Input: part model. Units: mm. Frame: model coordinates. Face numbers are marked on the shaded views. A direction names the side the tool comes from. Coordinates: 2 decimals unless noted, no trailing zeros. Loops run counter-clockwise (first coordinate to the right, second up) from the corner with the lowest first, then second, coordinate; pieces in that order, holes last. Notation, with made-up numbers: (74, -34) - (96, -34) arc R20 ccw to (96, -16) - close; hole circle Ø6 at (-19, 75.25). An arc over 180 degrees is marked (long way). Use a Markdown table: item, result. Add a question column.
1. Section query A-A on z = -7. Return the cut outline in (x, y), then the cut area to 3 significant figures.
2. Section query C-C on y = -7.5. Return the cut outline in (x, z).
3. Section query B-B on x = 4. Return the cut outline in (y, z).
4. Draft query along Y for the marked faces 3, 4 and 5. Return one class per face: released by +Y, released by -Y, zero draft, split by the parting line, or undercut.
5. Access query for the marked faces 1 and 2. Directions: +Z, -Z, +X, -X, +Y, -Y. A direction counts if a zero-diameter tool reaches every point of the face in a straight line with its end or side. Return the directions, or none.
6. Section query D-D on x = 16.5. Return the cut outline in (y, z), then the cut area to 3 significant figures.
7. Contact query for flat-ended pins moving along their axis: P1, Ø1.5, axis at x = 1, z = -3.5, coming from the -Y side; P2, Ø1.6, axis at x = 13.5, y = 2, coming from the +Z side; P3, Ø1.2, axis at x = 4, y = -47, coming from the +Z side. Output: stop coordinate, or through.
8. Ray query, L1, parallel to Y at x = 4, z = -4; L2, parallel to Y at x = 10.25, z = -4.5; L3, parallel to X at y = -47, z = -6. Return the intervals inside material, ascending. Write a range as [from, to].
Autodesk Inventor part; units mm, degrees
ref_plane "Płaszczyzna konstrukcyjna1" through (-42.5, -72.5, -8.25) normal (0, 0, 1) x (1, 0, 0)
ref_plane "YZ Plane" through (0, 0, 0) normal (1, 0, 0) x (0, 1, 0)
ref_plane "XZ Plane" through (0, 0, 0) normal (0, 1, 0) x (-1, 0, 0)
sketch "Szkic1" plane through (0, 0, 0) normal (0, 0, 1) x (1, 0, 0)
  line L0 (13.65, -45) -> (17, -45)
  line L1 (0.5, -45) -> (12.85, -45)
  line L2 (17, -25) -> (13.65, -25)
  line L3 (12.85, -25) -> (0.5, -25)
  line L4 (13.65, -20) -> (17, -20)
  line L5 (0.5, -20) -> (12.85, -20)
  line L6 (12.85, 0) -> (0.5, 0)
  line L7 (17, 0) -> (13.65, 0)
  line L8 (0, -25.5) -> (0, -44.5)
  line L9 (0, -0.5) -> (0, -19.5)
  line L10 (17.5, -12.6805) -> (17.5, -0.5)
  line L11 (17.5, -44.5) -> (17.5, -32.3195)
  line L12 (0, -45) -> (17.5, -45)
  line L13 (17.5, -45) -> (17.5, -49)
  line L14 (17.5, -49) -> (0, -49)
  line L15 (0, -49) -> (0, -45)
  line L16 (0, -20) -> (17.5, -20)
  line L17 (17.5, -20) -> (17.5, -25)
  line L18 (17.5, -25) -> (0, -25)
  line L19 (0, -25) -> (0, -20)
  line L20 (0, 0) -> (17.5, 0)
  line L21 (17.5, 0) -> (17.5, 4)
  line L22 (17.5, 4) -> (0, 4)
  line L23 (0, 4) -> (0, 0)
  line L24 (0, 4) -> (17.5, 4)
  line L25 (17.5, 4) -> (17.5, -49)
  line L26 (17.5, -49) -> (0, -49)
  line L27 (0, -49) -> (0, 4)
  dimension "d0" = 4
  dimension "d1" = 4
ref_plane "Płaszczyzna konstrukcyjna1" through (-42.5, -72.5, -8.25) normal (0, 0, 1) x (1, 0, 0)
extrude "Wyciągnięcie proste1" add sketch "Szkic1" against normal up to surface (8.25 mm away) contours L0 L12 L13 L14 L15 L1 | L18 L2 L3 L19 L16 L5 L4 L17 | L20 L7 L6 L23 L22 L21
sketch "Szkic2" plane through (0, 0, 0) normal (0, 0, 1) x (1, 0, 0)
  line L0 (0, 0) -> (17.5, 0)
  line L1 (17.5, 0) -> (17.5, 4)
  line L2 (17.5, 4) -> (0, 4)
  line L3 (0, 4) -> (0, 0)
  line L4 (0, -25) -> (17.5, -25)
  line L5 (17.5, -25) -> (17.5, -20)
  line L6 (17.5, -20) -> (0, -20)
  line L7 (0, -20) -> (0, -25)
  line L8 (0, -49) -> (17.5, -49)
  line L9 (17.5, -49) -> (17.5, -45)
  line L10 (17.5, -45) -> (0, -45)
  line L11 (0, -45) -> (0, -49)
  line L12 (0, 4) -> (17.5, 4)
  line L13 (17.5, 4) -> (0, 4)
  line L14 (0, 4) -> (0, -49)
  line L15 (0, -49) -> (17.5, -49)
  line L16 (17.5, -49) -> (17.5, 4)
extrude "Wyciągnięcie proste2" add sketch "Szkic2" along normal blind 2
sketch "Szkic3" plane through (0, 0, 2) normal (0, 0, 1) x (1, 0, 0)
  line L0 (17.5, -45) -> (0, -45)
  line L1 (0, 4) -> (0, -49)
  line L2 (0, -49) -> (17.5, -49)
  line L3 (17.5, -49) -> (17.5, 4)
  line L4 (0, -25) -> (17.5, -25)
  line L5 (17.5, -20) -> (0, -20)
  line L6 (0, 0) -> (17.5, 0)
  line L7 (17.5, 4) -> (0, 4)
  point P0 (13.5, -47)
  point P1 (4, -47)
  point P2 (13.5, -22.5)
  point P3 (4, -22.5)
  point P4 (13.5, 2)
  point P5 (4, 2)
  dimension "d6" = 2
  dimension "d7" = 2
  dimension "d8" = 2.5
  dimension "d9" = 2.5
  dimension "d10" = 2
  dimension "d11" = 2
  dimension "d12" = 4
  dimension "d13" = 4
  dimension "d14" = 4
  dimension "d15" = 4
  dimension "d16" = 4
  dimension "d17" = 4
hole "Otwór1" at (13.5, -47, 2) at (4, -47, 2) at (13.5, -22.5, 2) at (4, -22.5, 2) at (13.5, 2, 2) at (4, 2, 2) direction (0, 0, -1) diameter 2 end through all
sketch "Szkic4" plane through (0, 0, 2) normal (0, 0, 1) x (1, 0, 0)
  circle A0 centre (13.5, 2) radius 1
  circle A1 centre (13.5, -22.5) radius 1
  circle A2 centre (13.5, -47) radius 1
  circle A3 centre (4, -47) radius 1
  circle A4 centre (4, -22.5) radius 1
  circle A5 centre (4, 2) radius 1
  line L0 (17.5, -49) -> (17.5, 4)
  line L1 (17.5, 4) -> (0, 4)
  line L2 (0, 4) -> (0, -49)
  line L3 (0, -49) -> (17.5, -49)
  point P0 (0, 0)
extrude "Wyciągnięcie proste3" add sketch "Szkic4" against normal blind 3 contours A0 | A1 | A2 | A3 | A4 | A5
fillet "Zaokrąglenie1" radius 5 2 edges at (8.75, 4, 2) (8.75, -49, 2)
sketch "Szkic5" plane through (0, -25, -8.25) normal (-1, 0, 0) x (0, 0, 1)
  arc A0 (5.25, -24) -> (10.25, -19) centre (5.25, -19) ccw
  line L0 (10.25, 24) -> (10.25, -19)
  arc A1 (10.25, 24) -> (5.25, 29) centre (5.25, 24) ccw
  line L1 (0, 29) -> (5.25, 29)
  line L2 (0, 25) -> (0, 29)
  line L3 (8.25, 25) -> (0, 25)
  line L4 (8.25, 25) -> (8.25, 5)
  line L5 (8.25, 5) -> (0, 5)
  line L6 (0, 0) -> (0, 5)
  line L7 (8.25, 0) -> (0, 0)
  line L8 (8.25, 0) -> (8.25, -20)
  line L9 (8.25, -20) -> (0, -20)
  line L10 (0, -24) -> (0, -20)
  line L11 (5.25, -24) -> (0, -24)
  line L12 (0, 25) -> (0, -20)
extrude "Wyciągnięcie proste4" add sketch "Szkic5" along normal blind 1
fillet "Zaokrąglenie2" radius 4 5 edges at (-1, 4, -5.625) (-1, -22.5, 2) (-1, -47.5355, 0.5355) (-1, -49, -5.625) (-1, 2.5355, 0.5355)
sketch "Szkic6" plane through (17.5, -25, -8.25) normal (0, 0, -1) x (-1, 0, 0)
  circle A0 centre (13.5, -22) radius 1
  circle A1 centre (4, -22) radius 1
  circle A2 centre (13.5, 27) radius 1
  circle A3 centre (4, 27) radius 1
  circle A4 centre (4, 2.5) radius 1
  circle A5 centre (13.5, 2.5) radius 1
  arc A6 (18.5, 25) -> (14.5, 29) centre (14.5, 25) ccw
  line L0 (14.5, 29) -> (0, 29)
  line L1 (0, 29) -> (0, 25)
  line L2 (0, 25) -> (17.5, 25)
  line L3 (17.5, 25) -> (17.5, 5)
  line L4 (17.5, 5) -> (0, 5)
  line L5 (0, 5) -> (0, 0)
  line L6 (0, 0) -> (17.5, 0)
  line L7 (17.5, 0) -> (17.5, -20)
  line L8 (17.5, -20) -> (0, -20)
  line L9 (0, -20) -> (0, -24)
  line L10 (0, -24) -> (14.5, -24)
  arc A7 (14.5, -24) -> (18.5, -20) centre (14.5, -20) ccw
  line L11 (18.5, 25) -> (18.5, -20)
  line L12 (17.5, 0) -> (0, 0)
  line L13 (0, 5) -> (17.5, 5)
  line L14 (17.5, 5) -> (17.5, 0)
  line L15 (17.5, 0) -> (0, 0)
  line L16 (0, 0) -> (0, 5)
extrude "Wyciągnięcie proste5" cut sketch "Szkic6" against normal up to surface (8.25 mm away) contours A4 | A5 | L14 L6 L5 L4
properties part number "uchwyt_serw"
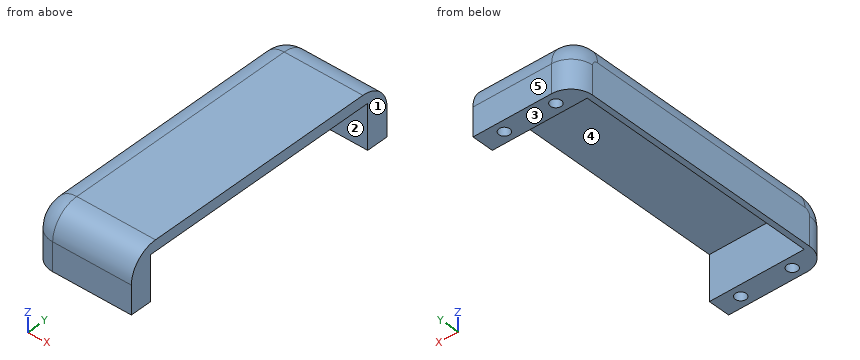
Resolved:
| question | item | result |
|---|---|---|
| 1 | outline | (-1, -45) arc R4 ccw to (3, -49) - (17.5, -49) - (17.5, -45) - (0, -45) - (0, 0) - (17.5, 0) - (17.5, 4) - (3, 4) arc R4 ccw to (-1, 0) - close; hole circle Ø2 at (4, -47); hole circle Ø2 at (4, 2); hole circle Ø2 at (13.5, -47); hole circle Ø2 at (13.5, 2) |
| 1 | area | 174 mm² |
| 2 | outline | (-1, -8.25) - (0, -8.25) - (0, 0) - (17.5, 0) - (17.5, 2) - (3, 2) arc R4 ccw to (-1, -2) - close |
| 3 | outline | (-49, -8.25) - (-48, -8.25) - (-48, -1) - (-46, -1) - (-46, -8.25) - (-45, -8.25) - (-45, 0) - (0, 0) - (0, -8.25) - (1, -8.25) - (1, -1) - (3, -1) - (3, -8.25) - (4, -8.25) - (4, -3) arc R5 ccw to (-1, 2) - (-44, 2) arc R5 ccw to (-49, -3) - close |
| 4 | face 3 | zero draft |
| 4 | face 4 | undercut |
| 4 | face 5 | released by +Y |
| 5 | face 1 | +Z, -Z, +X, +Y, -Y |
| 5 | face 2 | -Z, +X |
| 6 | outline | (-49, -8.25) - (-45, -8.25) - (-45, 0) - (0, 0) - (0, -8.25) - (4, -8.25) - (4, -3) arc R5 ccw to (-1, 2) - (-44, 2) arc R5 ccw to (-49, -3) - close |
| 6 | area | 161 mm² |
| 7 | P1 | y = -48.8 |
| 7 | P2 | z = 1.49 |
| 7 | P3 | z = 1.39 |
| 8 | L1 | [-49, -48], [-46, -45], [0, 1], [3, 4] |
| 8 | L2 | [-49, -45], [0, 4] |
| 8 | L3 | [-0.46, 3], [5, 12.5], [14.5, 17.5] |
